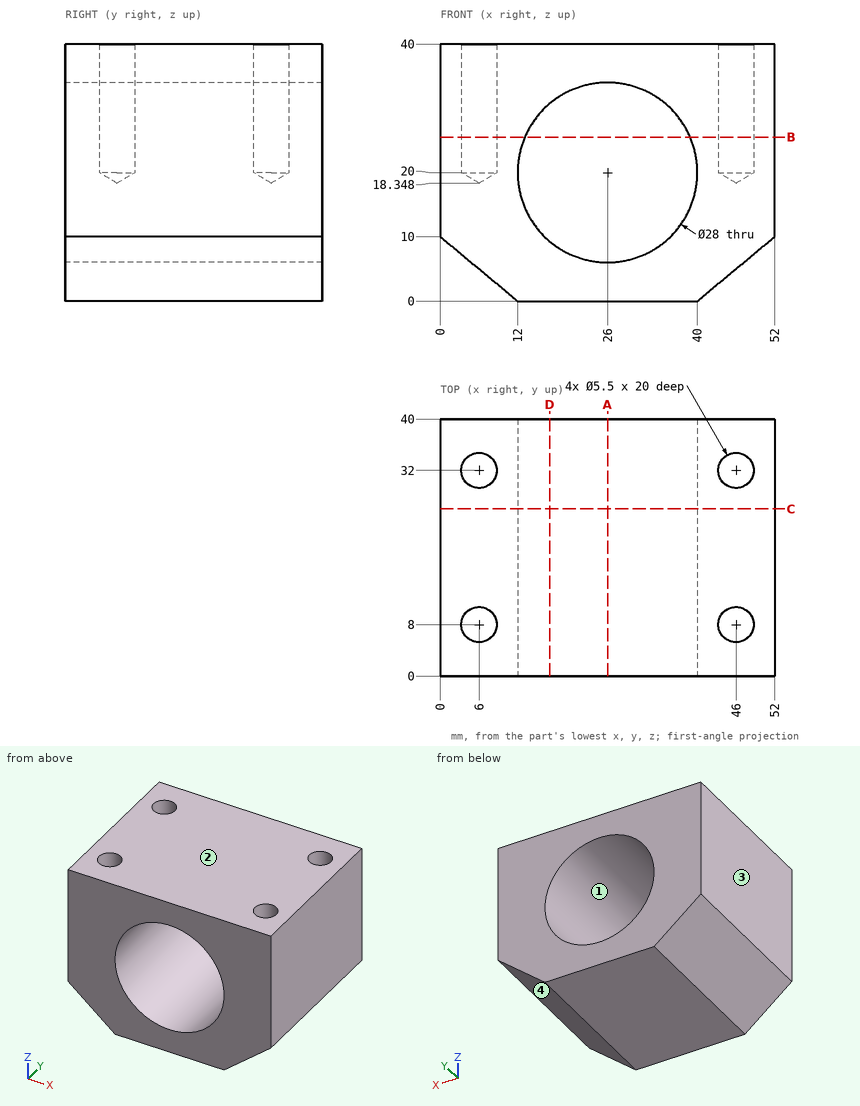
The drawing under review shows one solid part. Ordinate dimensions are in mm from its lowest x, y, z. Give positions to 0.01 mm unless a question says otherwise; leave off trailing zeros. Order: outer loops, then holes, each group sorted by start corner. A loop starts at its lowest first (then second) coordinate and runs counter-clockwise, first axis right, second up. Notation, with made-up numbers: (56, -8) - (110, -8) arc R9 ccw to (110, 7) - close; hole circle Ø9 at (88, 55). An arc over 180 degrees is marked (long way). Answer as a JSON object with one key per item and string values. Group by question number.
Item 1: Take a section at A-A on x = 26. Give the boundary of the cut face in (y, z).
Item 2: Draft analysis for pull direction Z (two halves, no side actions). For the marked faces 1, 2, 3 and 4, state which applies: pulls with the +Z half, pulls with the -Z half, needs draft (parallel to the pull), parting line crosses it, or undercut.
Item 3: Take a section at D-D on x = 17. Give the boundary of the cut face in (y, z).
Item 4: Take a section at B-B on z = 25.5. Give the number of separate pieces and of enclosed holes in the cut face, and give its area (3 significant figures).
Item 5: Clearance check with flat-ended pins moving along their axes: pin 1 Ø3.5 at (x, y) = (46, 32) entering from -Z; pin 2 Ø3.5 at (x, y) = (46, 8) entering from +Z; pin 3 Ø4.5 at (x, y) = (6, 32) entering from -Z (1 decimal). State where each tip first meets the part, or that it passes through.
Item 6: Take a section at C-C on y = 26. Give the boundary of the cut face in (x, z).
Item 7: Wall thickness on line 1 along X through (y, z) = (32, 35); line 2 along Y through (x, z) = (46, 33); line 3 along Z through (x, y) = (26, 18): over which ranges is each line inside the solid? List them lowest first.
Reported:
{
 "1": {"outline": "(0, 0) - (40, 0) - (40, 6) - (0, 6) - close; (0, 34) - (40, 34) - (40, 40) - (0, 40) - close"},
 "2": {"face 1": "undercut", "face 2": "pulls with the +Z half", "face 3": "needs draft", "face 4": "pulls with the -Z half"},
 "3": {"outline": "(0, 0) - (40, 0) - (40, 9.28) - (0, 9.28) - close; (0, 30.72) - (40, 30.72) - (40, 40) - (0, 40) - close"},
 "4": {"separate pieces": "2", "enclosed holes": "4", "area": "955 mm^2"},
 "5": {"pin 1": "z = 3.54", "pin 2": "z = 19.4", "pin 3": "z = 3.1"},
 "6": {"outline": "(0, 10) - (12, 0) - (40, 0) - (52, 10) - (52, 40) - (0, 40) - close; hole circle Ø28 at (26, 20)"},
 "7": {"line 1": "0 to 3.25, 8.75 to 43.25, 48.75 to 52", "line 2": "0 to 5.25, 10.75 to 29.25, 34.75 to 40", "line 3": "0 to 6, 34 to 40"}
}
